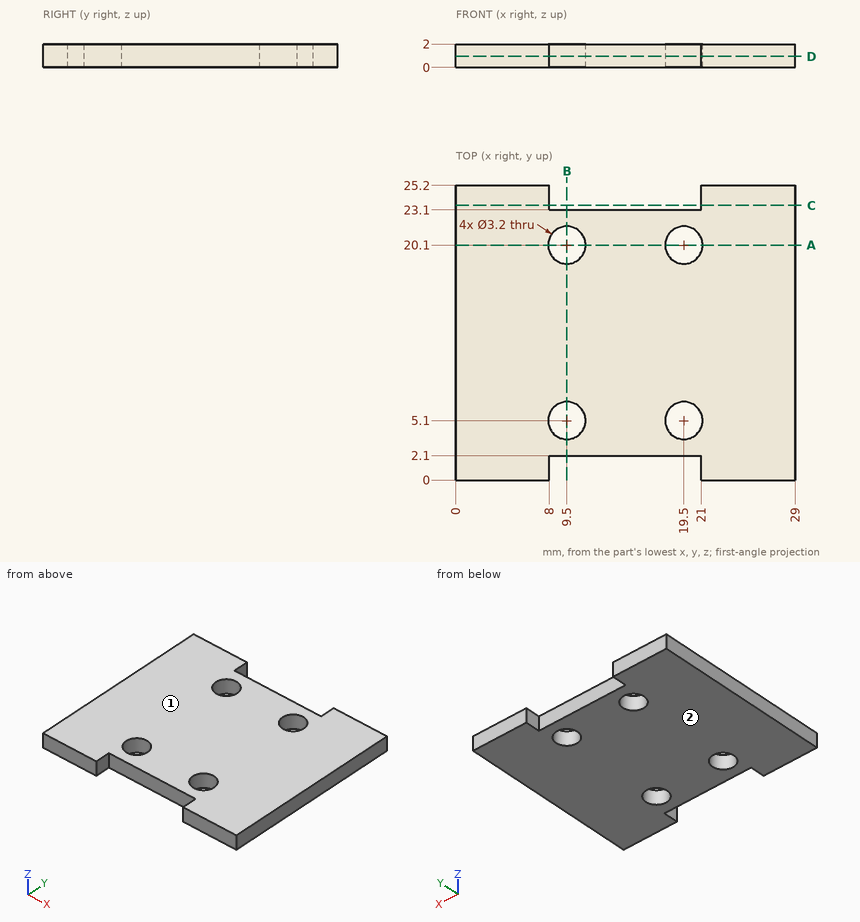
Part print with two shaded views. Sizes in mm from the minimum x, y, z corner. Round coordinates to 2 decimals unless told otherwise and drop trailing zeros. Write each loop counter-clockwise with the first axis right and the second up, starting at its lowest first coordinate (ties: lowest second). Pieces come first, ordered by that corner, then holes. Notation, with made-up numbers: M 85,89.25 L 94,89.25 A23 cw 94,107.25 Z; hole C -21,-20 d8. An arc over 180 degrees is marked long. Answer as CSV lines item,"result". Start each with the question number.
1) Drop flat-ended pins along their axis: pin 1 (3 mm diameter, centred on x = 9.5, y = 5.1, fed in from -Z); pin 2 (1 mm diameter, centred on x = 17, z = 0.5, fed in from +Y). Give the stop position or say it passes through.
2) Drill centre lines: L1, parallel to Y at x = 9.5, z = 0.4; L2, parallel to X at y = 5, z = 1.95; L3, parallel to Y at x = 20.5, z = 1.05. Where is each one in solid material? Low to high.
3) Band-saw the part on D-D (z = 0.95). List the corners of the cut face in (x, y).
4) Band-saw the part on A-A (y = 20.1). List the corners of the cut face in (x, z).
5) Band-saw the part on B-B (x = 9.5). List the corners of the cut face in (y, z).
6) Mould opens along Z. For the marked faces 1 and 2 say: +Z half, -Z half, draft (parallel to the pull), parting line (faces both ways), or undercut.
7) Band-saw the part on C-C (y = 23.5). List the corners of the cut face in (x, z), then the cut area to 3 significant figures.
Worked out:
1,pin 1,"through"
1,pin 2,"y = 23.1"
2,L1,"2.1 to 3.5, 6.7 to 18.5, 21.7 to 23.1"
2,L2,"0 to 7.9, 11.1 to 17.9, 21.1 to 29"
2,L3,"2.1 to 3.85, 6.35 to 18.85, 21.35 to 23.1"
3,outline,"M 0,0 L 8,0 L 8,2.1 L 21,2.1 L 21,0 L 29,0 L 29,25.2 L 21,25.2 L 21,23.1 L 8,23.1 L 8,25.2 L 0,25.2 Z; hole C 9.5,5.1 d3.2; hole C 9.5,20.1 d3.2; hole C 19.5,5.1 d3.2; hole C 19.5,20.1 d3.2"
4,outline,"M 0,0 L 7.9,0 L 7.9,2 L 0,2 Z; M 11.1,0 L 17.9,0 L 17.9,2 L 11.1,2 Z; M 21.1,0 L 29,0 L 29,2 L 21.1,2 Z"
5,outline,"M 2.1,0 L 3.5,0 L 3.5,2 L 2.1,2 Z; M 6.7,0 L 18.5,0 L 18.5,2 L 6.7,2 Z; M 21.7,0 L 23.1,0 L 23.1,2 L 21.7,2 Z"
6,face 1,"+Z half"
6,face 2,"-Z half"
7,outline,"M 0,0 L 8,0 L 8,2 L 0,2 Z; M 21,0 L 29,0 L 29,2 L 21,2 Z"
7,area,"32.0 mm²"
